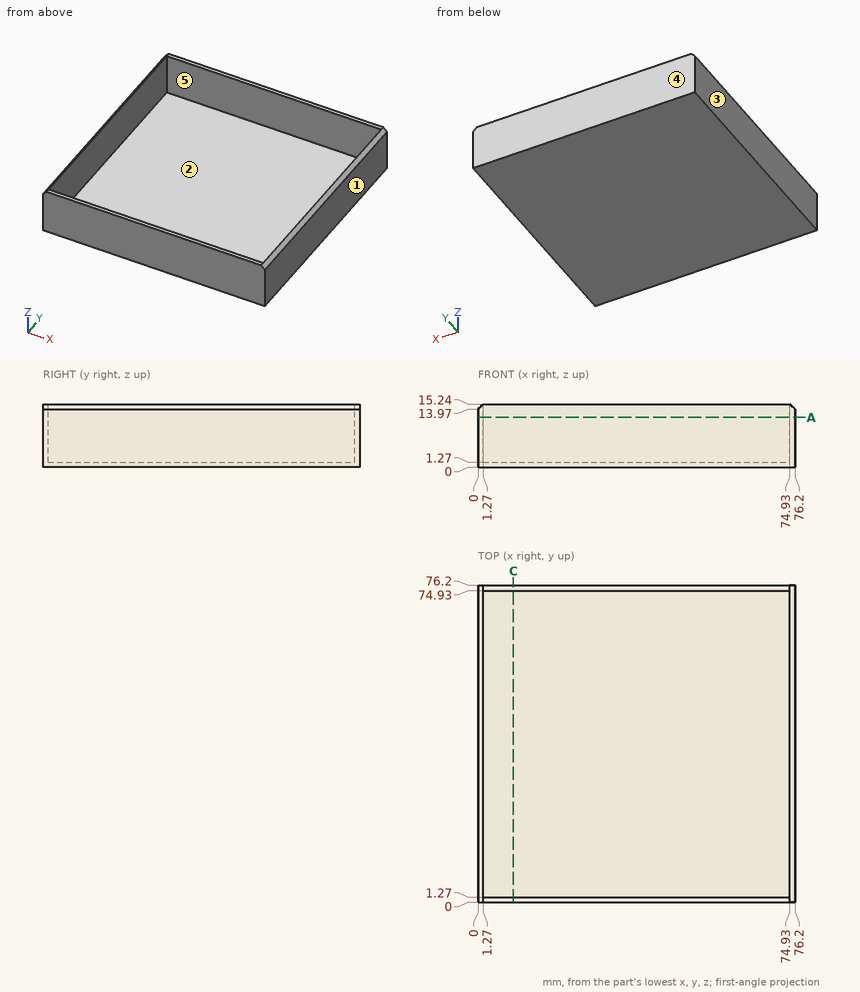
Can you work these out from the drawing? Everything is in mm from the part's minimum corner. A direction names the side the tool comes from. Give positions to 0.01 mm unless a question says otherwise; leave off trailing zeros. Loops run counter-clockwise (first coordinate to the right, second up) from the corner with the lowest first, then second, coordinate; pieces in that order, holes last. Notation, with made-up numbers: (-34.5, 63.25) - (-11.5, 63.25) arc R31 ccw to (-11.5, 97.25) - close; hole circle Ø10 at (26.5, 67). An arc over 180 degrees is marked (long way). Answer as a JSON object with one key per item and string values.
Q1. If I drill on L1, parallel to X at y = 15.5, z = 5; L2, parallel to Z at x = 33, y = 51.5, over which ranges is the centre line in solid material (lowest first)?
Geometry says:
{"L1": "0 to 1.27, 74.93 to 76.2", "L2": "0 to 1.27"}
Q2. Which directions (+Z, -Z, +X, -X, +Y, -Y) give clear straight access to the entire face, cutting with the end or side of a thin tool? Please do the marked faces 4 and 5.
Geometry says:
{"face 4": "+Z, -Z, +X, -X, +Y", "face 5": "+Z"}
Q3. Imagine slicing it at C-C on x = 8.5. Write out the boundary of the cut face in (y, z).
Geometry says:
{"outline": "(0, 0) - (76.2, 0) - (76.2, 15.24) - (74.93, 15.24) - (74.93, 1.27) - (1.27, 1.27) - (1.27, 15.24) - (0, 15.24) - close"}
Q4. Will this pin go through, and if not, where does the flat tip stop? P1, Ø5, axis at x = 29.5, y = 25.5, coming from the +Z side.
Geometry says:
{"P1": "z = 1.27"}
Q5. Imagine slicing it at A-A on z = 12. Write out the boundary of the cut face in (x, y), plus the area to 3 significant figures.
Geometry says:
{"outline": "(0, 0) - (76.2, 0) - (76.2, 76.2) - (0, 76.2) - close; hole (1.27, 1.27) - (74.93, 1.27) - (74.93, 74.93) - (1.27, 74.93) - close", "area": "381 mm²"}
Q6. If we mould it in two halves opening along X, with no side actions, what happens to the marked faces 1, 2 and 3? For each: pulls with the +X half, pulls with the -X half, needs draft (parallel to the pull), parting line crosses it, or undercut.
Geometry says:
{"face 1": "pulls with the +X half", "face 2": "undercut", "face 3": "pulls with the -X half"}
